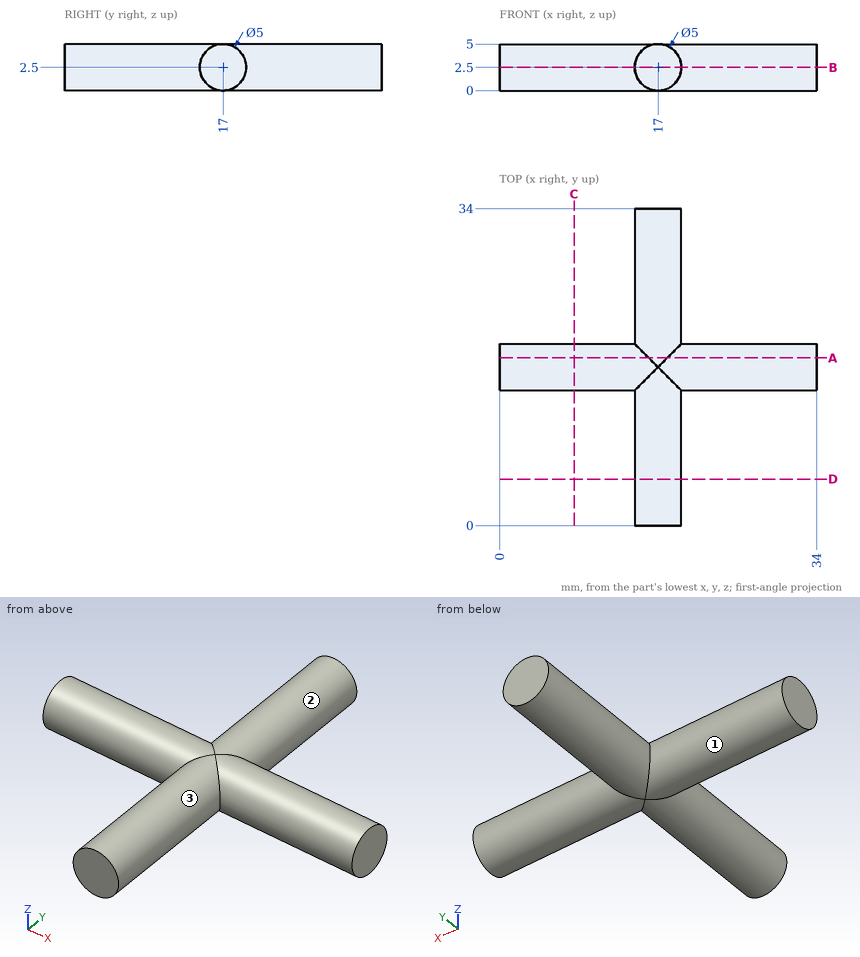
Design review of the part shown in the three views and the two pictorial views. Dimensions are in mm from the part's minimum x, y and z. A direction names the side the tool comes from. Coordinates: 2 decimals unless noted, no trailing zeros. Loops run counter-clockwise (first coordinate to the right, second up) from the corner with the lowest first, then second, coordinate; pieces in that order, holes last.
(1) Consider section B-B, the plane z = 2.5. Give the boundary of the cut face in (x, y), plus the area to 3 significant figures.
Determined:
outline: (0, 14.5) - (14.5, 14.5) - (14.5, 0) - (19.5, 0) - (19.5, 14.5) - (34, 14.5) - (34, 19.5) - (19.5, 19.5) - (19.5, 34) - (14.5, 34) - (14.5, 19.5) - (0, 19.5) - close
area: 315 mm2
(2) Insertion check: P1, Ø3, axis at x = 24.5, z = 2.5, coming from the -Y side; P2, Ø1.5, axis at x = 11.5, z = 4, coming from the -Y side; P3, Ø1, axis at y = 26.5, z = 4, coming from the +X side. Each pin has a flat end and moves straight along its axis. Give the tip position at first contact, or say it passes through.
Determined:
P1: stops at y = 14.5
P2: stops at y = 14.62
P3: stops at x = 19.29
(3) Wall thickness on L1, parallel to Y at x = 23, z = 2.5; L2, parallel to X at y = 10, z = 3.75: over which ranges is each line inside the solid? List them lowest first.
Determined:
L1: y = 14.5 to 19.5
L2: x = 14.83 to 19.17
(4) Consider section A-A, the plane y = 18. Give the boundary of the cut face in (x, z).
Determined:
outline: (0, 0.21) - (16, 0.21) arc R2.5 ccw to (18, 0.21) - (34, 0.21) - (34, 4.79) - (18, 4.79) arc R2.5 ccw to (16, 4.79) - (0, 4.79) - close
(5) Tool access review of the marked faces 1, 2 and 3: name each direction out of +Z, -Z, +X, -X, +Y, -Y from which nothing blocks a thin tool from reaching the whole face with its end or side.
Determined:
face 1: -X
face 2: +Y
face 3: -Y
(6) Consider section C-C, the plane x = 8. Give the boundary of the cut face in (y, z), plus the area to 3 significant figures.
Determined:
outline: circle Ø5 at (17, 2.5)
area: 19.6 mm2
